```python
from build123d import *

# Parameters (mm, degrees)
SKETCH1_R                    = 15.875
SKETCH1_R_2                  = 14.2875
BOSS_EXTRUDE1_DEPTH          = 1739.9
F_10_0_1935_DIAMETER_HOLE1_D = 4.9149
F_10_0_1935_DIAMETER_HOLE2_D = 4.9149


with BuildPart() as part:
    # Sketch1 → Boss-Extrude1 (new body)
    with BuildSketch(Plane.XY):
        Circle(SKETCH1_R)
        Circle(SKETCH1_R_2, mode=Mode.SUBTRACT)
    extrude(amount=BOSS_EXTRUDE1_DEPTH)

    # #10 (0.1935) Diameter Hole1 (through all)
    with Locations(Plane(origin=(0, -15.875, 6.35), x_dir=(-1, 0, 0), z_dir=(0, -1, 0))):
        with Locations((0, 0)):
            Hole(F_10_0_1935_DIAMETER_HOLE1_D / 2)

    # #10 (0.1935) Diameter Hole2 (through all)
    with Locations(Plane(origin=(0, 15.875, 1733.55), x_dir=(1, 0, 0), z_dir=(0, 1, 0))):
        with Locations((0, 0)):
            Hole(F_10_0_1935_DIAMETER_HOLE2_D / 2)


solid = part.part
```
Design review of the part built by this model. Coordinates are the model's own, in mm. Give positions to 0.01 mm unless a question says otherwise; leave off trailing zeros. Order: outer loops, then holes, each group sorted by start corner. A loop starts at its lowest first (then second) coordinate and runs counter-clockwise, first axis right, second up. Notation, with made-up numbers: (32.25, 80.5) - (37.25, 80.5) arc R8 ccw to (37.25, 90.5) - close; hole circle Ø11 at (67.25, 87.5). An arc over 180 degrees is marked (long way). Use a Markdown table: item, result. Add a question column.
(1) Mouldability with a two-part tool opening along X and no side actions: class faces 1 (the face through (-3.441, -15.497, 857.771)), 2 (the face through (-14.274, 0.628, 857.771)), 3 (the face through (-11.83, 8.31, 1739.9)) as +X half, -X half, draft (parallel to the pull), parting line (faces both ways), or undercut.
(2) Clearance check with flat-ended pins moving along their axes: P1, Ø10, axis at x = 5.5, z = 1098.5, coming from the +Y side; P2, Ø1, axis at x = 7.5, z = 1492, coming from the +Y side; P3, Ø2, axis at y = 8, z = 1374, coming from the -X side. State where each tip first meets the part, or that it passes through.
(3) Wall thickness on probe 1 along Z at (x, y) = (0, -15.45); probe 2 along X at (y, z) = (-0.5, 1532); probe 3 along X at (y, z) = (1, 169): over which ranges is each line inside the solid? List them lowest first. Write a range as [from, to].
(4) Add section A-A on y = 0. Give the boundary of the cut face in (x, z) (1 decimal).
Report:
| question | item | result |
|---|---|---|
| 1 | face 1 | parting line |
| 1 | face 2 | undercut |
| 1 | face 3 | draft |
| 2 | P1 | stops at y = 15.87 |
| 2 | P2 | stops at y = 14.25 |
| 2 | P3 | stops at x = -14.25 |
| 3 | probe 1 | z = [0, 3.89], [8.81, 1731.09], [1736.01, 1739.9] |
| 3 | probe 2 | x = [-15.87, -14.28], [14.28, 15.87] |
| 3 | probe 3 | x = [-15.84, -14.25], [14.25, 15.84] |
| 4 | outline | (-15.9, 0) - (-14.3, 0) - (-14.3, 1739.9) - (-15.9, 1739.9) - close; (14.3, 0) - (15.9, 0) - (15.9, 1739.9) - (14.3, 1739.9) - close |
